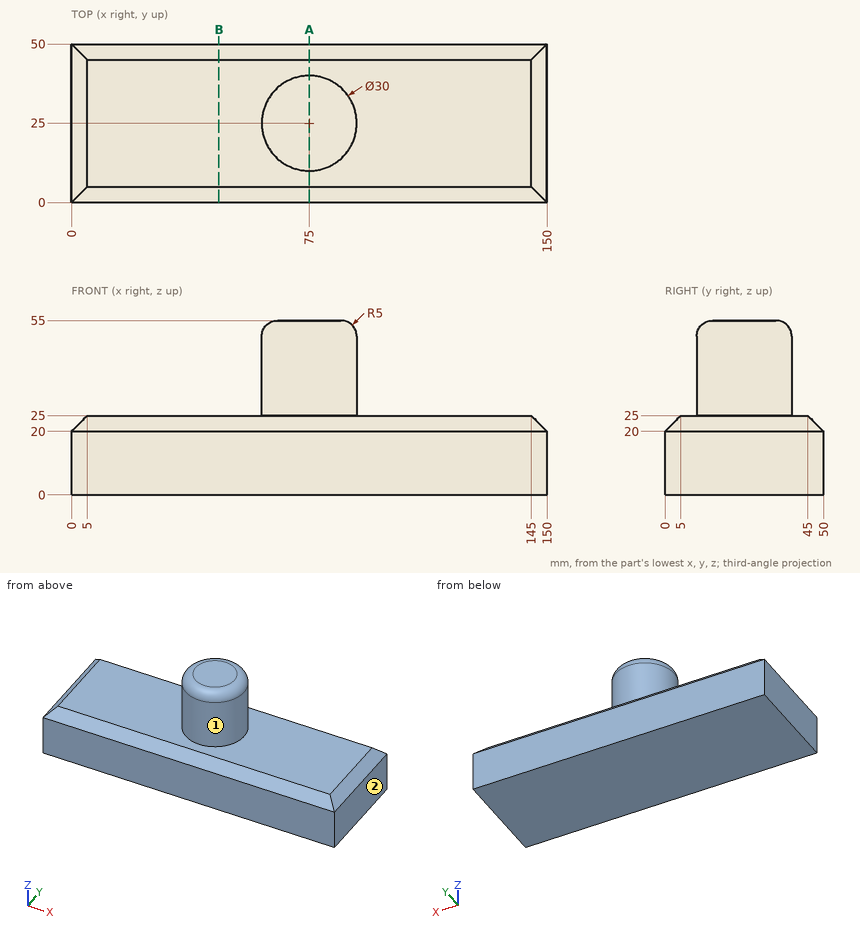
Source: three-view drawing plus pictorial views. Frame: mm from the lowest corner of the part. A direction names the side the tool comes from. Coordinates: 2 decimals unless noted, no trailing zeros. Order: outer loops, then holes, each group sorted by start corner. A loop starts at its lowest first (then second) coordinate and runs counter-clockwise, first axis right, second up.
Item 1: First-contact query: P1, Ø12, axis at x = 94, y = 12.5, coming from the +Z side; P2, Ø2, axis at y = 7.5, z = 42.5, coming from the -X side; P3, Ø6, axis at y = 31.5, z = 49, coming from the +X side; P4, Ø4, axis at y = 17.5, z = 27.5, coming from the -X side. Flat tips, straight axial feed; report the tip coordinate or a pass-through.
Output values:
P1: stops at z = 25
P2: passes through
P3: stops at x = 89.59
P4: stops at x = 61.04
Item 2: Cut plane B-B (x = 46.5). Return loops of the section in (y, z), plus the area to 4 significant figures.
Output values:
outline: (0, 0) - (50, 0) - (50, 20) - (45, 25) - (5, 25) - (0, 20) - close
area: 1,225 mm2
Item 3: Set-up query: the marked faces 1 and 2. Return all of +Z, -Z, +X, -X, +Y, -Y with unobstructed straight access to the full face (end or side cutting, diameter ignored); none if empty.
Output values:
face 1: +Z
face 2: +Z, -Z, +X, +Y, -Y
Item 4: Material intervals for line 1 (Z direction, x = 99.5, y = 37); line 2 (X direction, y = 25, z = 23); line 3 (X direction, y = 23, z = 49), sorted ascending.
Output values:
line 1: z = 0 to 25
line 2: x = 3 to 147
line 3: x = 60.13 to 89.87
Item 5: Cut plane A-A (x = 75). Return loops of the section in (y, z).
Output values:
outline: (0, 0) - (50, 0) - (50, 20) - (45, 25) - (40, 25) - (40, 50) arc R5 ccw to (35, 55) - (15, 55) arc R5 ccw to (10, 50) - (10, 25) - (5, 25) - (0, 20) - close
